Read the model definition and answer for the solid it produces. Units are mm, in the model's axes. Face numbers are marked on the shaded views. A direction names the side the tool comes from. Round coordinates to 2 decimals unless told otherwise and drop trailing zeros. Loops run counter-clockwise (first coordinate to the right, second up) from the corner with the lowest first, then second, coordinate; pieces in that order, holes last. Notation, with made-up numbers: (12.25, -33.75) -> (44.25, -33.75) arc R20 cw to (44.25, -5.75) -> close; hole circle Ø1 at (85.25, 5.25). An arc over 180 degrees is marked (long way). Put each result on its own line as item: value.
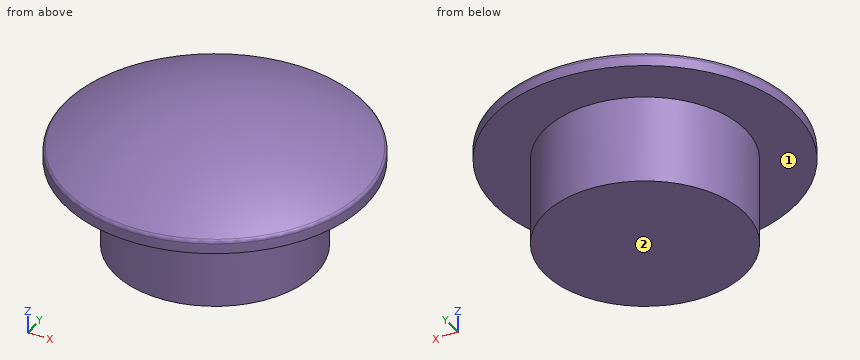
from build123d import *

# Parameters (mm, degrees)
F0_R     = 6.35
F1_DEPTH = 3.175
F4_R     = 0.254


with BuildPart() as f1:
    # F0 (on Top) → F1 (new body, symmetric)
    with BuildSketch(Plane.XY):
        Circle(F0_R)
    extrude(amount=F1_DEPTH, both=True)

    # F2 (on Front) → F3 (revolve)
    with BuildSketch(Plane.XZ):
        with BuildLine():
            Line((9.525, 2.38125), (9.525, 3.175))
            ThreePointArc((9.525, 3.175), (4.930503, 5.078103), (0, 5.727216))
            Line((0, 5.727216), (0, 2.38125))
            Line((0, 2.38125), (9.525, 2.38125))
        make_face()
    revolve(axis=Axis((0, 0, 4.054233), (0, 0, 1)))

    # F4
    f4_edges = [f1.edges().sort_by_distance(p)[0] for p in [
        (-9.525, 0, 3.175),
    ]]
    fillet(f4_edges, radius=F4_R)


solid = f1.part
Item 1: The part is cut by section A-A (z = 1). Determine the outline of the cut face in (x, y), then the cut area to 3 significant figures.
Derived:
outline: circle Ø12.7 at (0, 0)
area: 127 mm^2
Item 2: Flat-ended cylindrical pins translate along their axes: pin 1 Ø1 at (y, z) = (-4.5, 0.5) entering from +X; pin 2 Ø1 at (x, y) = (4, -7) entering from +Z; pin 3 Ø2 at (x, y) = (-2.5, -5) entering from +Z. Find the tip coordinate at first contact, or state that the pin passes through.
Derived:
pin 1: stops at x = 4.93
pin 2: stops at z = 4.16
pin 3: stops at z = 5.17
Item 3: Find the intervals of material crossed by line 1 along Y through (x, z) = (-0.25, -0.5); line 2 along Z through (x, y) = (3.25, -5) (3 decimals); line 3 along Z through (x, y) = (2.5, -6.5), in increasing order.
Derived:
line 1: y = -6.35 to 6.35
line 2: z = -3.175 to 4.77
line 3: z = 2.38 to 4.41
Item 4: Which of the six approach directions +Z, -Z, +X, -X, +Y, -Y give full straight-line access (tool end or side, diameter ignored) to the marked faces 1 and 2?
Derived:
face 1: -Z
face 2: -Z, +X, -X, +Y, -Y
